from build123d import *

# Parameters (mm, degrees)
SKETCH_1_R        = 0.9
EXTRUDE_1_DEPTH   = 3.5
SWEEP_1_PROFILE_R = 0.75
FILLET_2_R        = 1


with BuildPart() as part:
    # 草图1 → 凸台-拉伸1 (new body)
    with BuildSketch(Plane(origin=(0, 0, 0), x_dir=(1, 0, 0), z_dir=(0, 1, 0))):
        with Locations(Location((0, 0, 0), (0, 0, 270))):
            Circle(SKETCH_1_R)
    extrude(amount=EXTRUDE_1_DEPTH)

    # 扫描1: sweep along a path in 草图2
    with BuildLine(Plane(origin=(0, 0, 0), x_dir=(0, 0, -1), z_dir=(1, 0, 0))) as sweep_1_path:
        Line((6.840402867, 35.793852416), (0.603073792, 18.656931626))
        ThreePointArc((0.603073792, 18.656931626), (0.15192247, 16.97321197), (0, 15.236730193))
        Line((0, 15.236730193), (0, 3))
    # 扫描1 profile (on start of the path) → 扫描1 (sweep)
    with BuildSketch(Plane(origin=(0, 35.793852416, -6.840402867), x_dir=(0, -0.34202014332566616, -0.9396926207859094), z_dir=(0, -0.9396926207859094, 0.34202014332566616))):
        Circle(SWEEP_1_PROFILE_R)
    sweep(path=sweep_1_path.line)

    # 草图20 one side → 旋转7 (revolve)
    with BuildSketch(Plane(origin=(0, 33.805230182, -12.304097549), x_dir=(1, 0, 0), z_dir=(0, 0.9396926207859094, -0.3420201433256662))):
        with BuildLine():
            ThreePointArc((-1.5, -5.814342437), (0, -7.314342437), (1.5, -5.814342437))
            Line((1.5, -5.814342437), (0.75, -5.814342437))
            ThreePointArc((0.75, -5.814342437), (0, -6.564342437), (-0.75, -5.814342437))
            Line((-0.75, -5.814342437), (-1.5, -5.814342437))
        make_face()
    revolve(axis=Axis((0, 35.793852416, -6.840402867), (-1, 0, 0)))

    # 圆角2
    # the kernel refuses this fillet: 1 mm, written as the material it adds along each edge
    with BuildSketch(Plane(origin=(0, 3.5, 0), x_dir=(0, 0, -1), z_dir=(-1, 0, 0))) as fillet_2_piece_1:
        with BuildLine():
            CenterArc((1.75, -0.526782688), FILLET_2_R, 148.211669382, 31.788330618)
            Line((0.75, -0.526782688), (0.73, -0.526782688))
            Line((0.73, -0.526782688), (0.73, 0))
            Line((0.73, 0), (0.75, 0.02))
            ThreePointArc((0.75, 0.02), (0.825, 0.02), (0.883, 0.010535654))
            Line((0.883, 0.010535654), (0.9, 0))
        make_face()
    revolve(axis=Axis((0, 3.5, 0), (0, -1, 0)))


solid = part.part
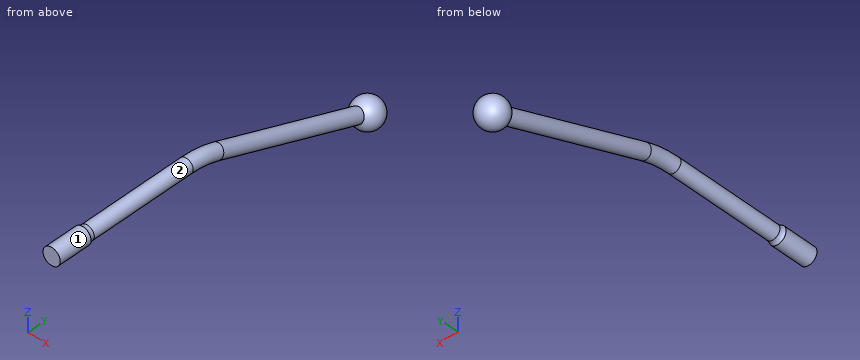
Can you work these out from the model? Positions are in its coordinate system, mm. Face numbers are marked on the shaded views. Give positions to 0.01 mm unless a question says otherwise; leave off trailing zeros. Order: outer loops, then holes, each group sorted by start corner. A loop starts at its lowest first (then second) coordinate and runs counter-clockwise, first axis right, second up. Notation, with made-up numbers: M 17,49 L 44,49 A20 ccw 44,65 Z; hole C 70,44 d5. An arc over 180 degrees is marked long. Use one line per item in the form item = value. Start each with the question number.
Item 1: If we section it at B-B (y = 9): Write out the boundary of the cut face in (x, z), then the cut area to 3 significant figures.
Item 2: If I drill on line 1 along Z through (x, y) = (-0.2, 26); line 2 along Y through (x, z) = (0.9, -7.5); line 3 along Y through (x, z) = (0.8, -7.5), over which ranges is the centre line in solid material (lowest first)?
Item 3: We'd pull the mould along Y, two halves only. Please class the marked faces 1 and 2: +Y half, -Y half, draft (parallel to the pull), parting line (faces both ways), or undercut.
Item 4: If we section it at A-A (x = 0): Write out the boundary of the cut face in (y, z), then the cut area to 3 significant figures.
Item 5: Will this pin go through, and if not, where does the flat tip stop? pin 1 Ø4 at (y, z) = (13, -1.5) entering from +X.
Outcome:
q1.outline = C 0,0 d1.5
q1.area = 1.77 mm2
q2.line_1 = -4.04 to -2.51
q2.line_2 = 34.79 to 36.8
q2.line_3 = 34.71 to 36.88
q3.face_1 = draft
q3.face_2 = undercut
q4.outline = M 0,-0.9 L 3.5,-0.9 A1 cw 4.03,-0.75 L 15.24,-0.75 A9.25 cw 18.4,-1.31 L 34.32,-7.1 A1.5 ccw long 34.83,-5.69 L 18.91,0.1 A10.75 ccw 15.24,0.75 L 4.03,0.75 A1 cw 3.5,0.9 L 0,0.9 Z; hole M 35.54,-7.55 A0.75 ccw 36.05,-6.14 Z
q4.area = 60.6 mm2
q5.pin_1 = 0.75
